Design review of the part built by this model. Coordinates are the model's own, in mm. Face numbers are marked on the shaded views. A direction names the side the tool comes from. Coordinates: 2 decimals unless noted, no trailing zeros. Write each loop counter-clockwise with the first axis right and the second up, starting at its lowest first coordinate (ties: lowest second). Pieces come first, ordered by that corner, then holes.
```python
from build123d import *

# Parameters (mm, degrees)
F0_W     = 19
F0_H     = 9
F1_DEPTH = 5
F2_DEPTH = 5


with BuildPart() as f1:
    # F0 (on Top) → F1 (new body)
    with BuildSketch(Plane.XY):
        Polygon((23, -4), (23, 0), (23, 13), (-4, 13), (-4, -4), align=None)
        with Locations((9.5, 4.5)):
            Rectangle(F0_W, F0_H, mode=Mode.SUBTRACT)
        with Locations((9.5, 4.5)):
            Rectangle(F0_W, F0_H)
    extrude(amount=-F1_DEPTH)

    # F0 (on Top) → F2 (join)
    with BuildSketch(Plane.XY):
        Polygon((23, -4), (23, 0), (23, 13), (-4, 13), (-4, -4), align=None)
        with Locations((9.5, 4.5)):
            Rectangle(F0_W, F0_H, mode=Mode.SUBTRACT)
    extrude(amount=F2_DEPTH)


solid = f1.part
```
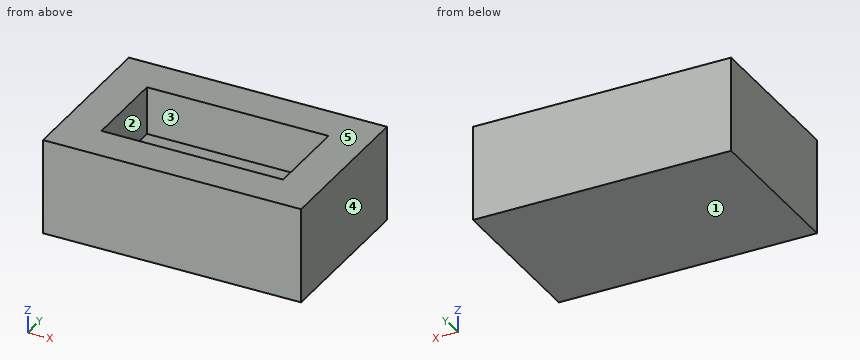
(1) Consider section A-A (z = 0.5). Give the boundary of the cut face in (x, y).
(2) Consider section B-B (x = 14.5). Give the boundary of the cut face in (y, z), plus the area to 3 significant figures.
(3) For the marked faces 1 and 2, list the 3-axis set-ups (+Z, -Z, +X, -X, +Y, -Y) from which the entire face can be reached by the end or side of a thin tool; tool diameter is ignored.
(4) Mouldability with a two-part tool opening along X and no side actions: class the marked faces 3, 4 and 5 as +X half, -X half, draft (parallel to the pull), parting line (faces both ways), or undercut.
(5) Consider section C-C (y = 5.75). Give the boundary of the cut face in (x, z).
(6) Wall thickness on line 1 (Y direction, x = 11.75, z = 3.5); line 2 (X direction, y = 3, z = 3.5); line 3 (Z direction, x = 11.75, y = 3.75): over which ranges is each line inside the solid? List them lowest first.
(7) Insertion check: pin 1 Ø1.5 at (x, y) = (14, 3) entering from +Z. The pin has a flat end and moves straight along its axis. Give the tip position at first contact, or say it passes through.
Results:
1. outline: (-4, -4) - (23, -4) - (23, 13) - (-4, 13) - close; hole (0, 0) - (19, 0) - (19, 9) - (0, 9) - close
2. outline: (-4, -5) - (13, -5) - (13, 5) - (9, 5) - (9, 0) - (0, 0) - (0, 5) - (-4, 5) - close
2. area: 125 mm2
3. face 1: -Z, +X, -X, +Y, -Y
3. face 2: +Z
4. face 3: undercut
4. face 4: +X half
4. face 5: draft
5. outline: (-4, -5) - (23, -5) - (23, 5) - (19, 5) - (19, 0) - (0, 0) - (0, 5) - (-4, 5) - close
6. line 1: y = -4 to 0, 9 to 13
6. line 2: x = -4 to 0, 19 to 23
6. line 3: z = -5 to 0
7. pin 1: stops at z = 0
